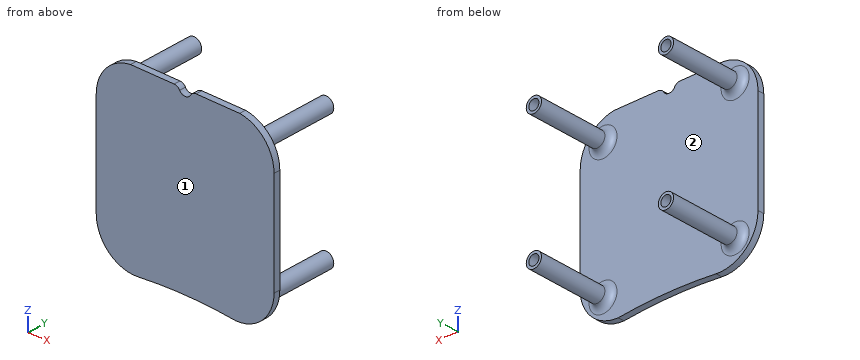
```python
from build123d import *

# Parameters (mm, degrees)
BOSS_EXTRUDE1_DEPTH = 5
SKETCH3_R           = 6
SKETCH3_R_2         = 2
BOSS_EXTRUDE2_DEPTH = 60
SKETCH4_R           = 4
CUT_EXTRUDE2_DEPTH  = 20
FILLET1_R           = 5
SKETCH5_R           = 5
CUT_EXTRUDE3_DEPTH  = 10
FILLET2_R           = 5


with BuildPart() as part:
    # Sketch2 → Boss-Extrude1 (new body)
    with BuildSketch(Plane(origin=(0, 0, 0), x_dir=(1, 0, 0), z_dir=(0, 1, 0))):
        with BuildLine():
            Line((-53.508823352, -72.096737708), (32.436645713, -72.096737708))
            ThreePointArc((32.436645713, -72.096737708), (51.703313555, -62.379157363), (59.46391118, -42.24438689))
            Line((59.46391118, -42.24438689), (59.46391118, 38.050911473))
            ThreePointArc((59.46391118, 38.050911473), (50.695521882, 59.245691656), (29.51599738, 68.050866257))
            ThreePointArc((29.51599738, 68.050866257), (-9.019885151, 65.996186888), (-47.563354288, 67.903262292))
            ThreePointArc((-47.563354288, 67.903262292), (-70.670859293, 60.290313848), (-80.53608882, 38.050911473))
            Line((-80.53608882, 38.050911473), (-80.53608882, -42.24438689))
            ThreePointArc((-80.53608882, -42.24438689), (-72.775491194, -62.379157363), (-53.508823352, -72.096737708))
        make_face()
    extrude(amount=BOSS_EXTRUDE1_DEPTH)

    # Sketch3 → Boss-Extrude2 (add)
    # profile 1 of 4: a face of its own
    with BuildSketch(Plane(origin=(0, 5, 0), x_dir=(1, 0, 0), z_dir=(0, 1, 0))):
        with Locations(Location((41.46391118, 49.903262292, 0), (0, 0, 90))):
            Circle(SKETCH3_R)
        with Locations(Location((41.46391118, 49.903262292, 0), (0, 0, 270))):
            Circle(SKETCH3_R_2, mode=Mode.SUBTRACT)
    # profile 2 of 4: a face of its own
    with BuildSketch(Plane(origin=(0, 5, 0), x_dir=(1, 0, 0), z_dir=(0, 1, 0))):
        with Locations(Location((-62.53608882, 49.903262292, 0), (0, 0, 90))):
            Circle(SKETCH3_R)
        with Locations(Location((-62.53608882, 49.903262292, 0), (0, 0, 90))):
            Circle(SKETCH3_R_2, mode=Mode.SUBTRACT)
    # profile 3 of 4: a face of its own
    with BuildSketch(Plane(origin=(0, 5, 0), x_dir=(1, 0, 0), z_dir=(0, 1, 0))):
        with Locations(Location((-62.53608882, -54.096737708, 0), (0, 0, 90))):
            Circle(SKETCH3_R)
        with Locations(Location((-62.53608882, -54.096737708, 0), (0, 0, 270))):
            Circle(SKETCH3_R_2, mode=Mode.SUBTRACT)
    # profile 4 of 4: a face of its own
    with BuildSketch(Plane(origin=(0, 5, 0), x_dir=(1, 0, 0), z_dir=(0, 1, 0))):
        with Locations(Location((41.46391118, -54.096737708, 0), (0, 0, 90))):
            Circle(SKETCH3_R)
        with Locations(Location((41.46391118, -54.096737708, 0), (0, 0, 90))):
            Circle(SKETCH3_R_2, mode=Mode.SUBTRACT)
    extrude(amount=BOSS_EXTRUDE2_DEPTH)

    # Sketch4 → Cut-Extrude2 (cut)
    with BuildSketch(Plane(origin=(0, 65, 0), x_dir=(1, 0, 0), z_dir=(0, 1, 0))):
        with Locations(Location((41.46391118, 49.903262292, 0), (0, 0, 270))):
            Circle(SKETCH4_R)
        with Locations(Location((-62.53608882, 49.903262292, 0), (0, 0, 270))):
            Circle(SKETCH4_R)
        with Locations(Location((-62.53608882, -54.096737708, 0), (0, 0, 270))):
            Circle(SKETCH4_R)
        with Locations(Location((41.46391118, -54.096737708, 0), (0, 0, 270))):
            Circle(SKETCH4_R)
    extrude(amount=-CUT_EXTRUDE2_DEPTH, mode=Mode.SUBTRACT)

    # Fillet1
    fillet1_edges = [part.edges().sort_by_distance(p)[0] for p in [
        (41.46391118, 5, -43.903262292),
        (-62.53608882, 5, -43.903262292),
        (-62.53608882, 5, 60.096737708),
        (41.46391118, 5, 60.096737708),
    ]]
    fillet(fillet1_edges, radius=FILLET1_R)

    # Sketch5 → Cut-Extrude3 (cut)
    with BuildSketch(Plane(origin=(0, 5, 0), x_dir=(1, 0, 0), z_dir=(0, 1, 0))):
        with Locations((-10.53608882, -72.096737708)):
            Circle(SKETCH5_R)
    extrude(amount=-CUT_EXTRUDE3_DEPTH, mode=Mode.SUBTRACT)

    # Fillet2
    fillet2_edges = [part.edges().sort_by_distance(p)[0] for p in [
        (-15.53608882, 2.5, 72.096737708),
        (-5.53608882, 2.5, 72.096737708),
    ]]
    fillet(fillet2_edges, radius=FILLET2_R)


solid = part.part
```
Design review of the part built by this model. Coordinates are the model's own, in mm. Face numbers are marked on the shaded views. Give positions to 0.01 mm unless a question says otherwise; leave off trailing zeros. Order: outer loops, then holes, each group sorted by start corner. A loop starts at its lowest first (then second) coordinate and runs counter-clockwise, first axis right, second up. Notation, with made-up numbers: (81.5, 60) -> (93.5, 60) arc R13 ccw to (93.5, 77) -> close; hole circle Ø10 at (-7.5, 62.5). An arc over 180 degrees is marked (long way). Write each question's results on one line, items separated by ' | '. Start each with the question number.
Q1. Wall thickness on L1, parallel to X at y = 11.5, z = -50; L2, parallel to X at y = 16.5, z = 53 (3 decimals); L3, parallel to Y at x = 27, z = -41: over which ranges is each line inside the solid? List them lowest first. Write a range as from..to.
Q2. Add section D-D on x = -44. Give the boundary of the cut face in (y, z), and give its area (3 significant figures).
Q3. For pin 1 (2 mm diameter, centred on y = 7.5, z = -15, fed in from -X); pin 2 (8 mm diameter, centred on x = -40, z = -29.5, fed in from +Y); pin 3 (3 mm diameter, centred on x = 40.5, z = -51, fed in from +Y), all flat-tipped, find the tip position at first contact; note any pin that passes through.
Q4. Add section B-B on y = 47.5. Give the boundary of the cut face in (x, z).
Q5. Add section A-A on y = 38. Give the boundary of the cut face in (x, z), and give its area (3 significant figures).
Q6. Add section C-C on z = 15. Give the boundary of the cut face in (x, y).
Q7. Mouldability with a two-part tool opening along X and no side actions: class the marked faces 1 and 2 as +X half, -X half, draft (parallel to the pull), parting line (faces both ways), or undercut.
Found:
1) L1: x = -68.54..-64.53, -60.54..-56.54, 35.46..39.47, 43.46..47.46 | L2: x = -68.435..-64.209, -60.864..-56.637, 35.565..39.791, 43.136..47.363 | L3: y = 0..5
2) outline: (0, -67.56) -> (5, -67.56) -> (5, 72.1) -> (0, 72.1) -> close | area: 698 mm2
3) pin 1: passes through | pin 2: stops at y = 5 | pin 3: stops at y = 45
4) outline: circle Ø12 at (-62.54, -49.9); circle Ø12 at (-62.54, 54.1); circle Ø12 at (41.46, -49.9); circle Ø12 at (41.46, 54.1); hole circle Ø8 at (-62.54, -49.9); hole circle Ø8 at (-62.54, 54.1); hole circle Ø8 at (41.46, -49.9); hole circle Ø8 at (41.46, 54.1)
5) outline: circle Ø12 at (-62.54, -49.9); circle Ø12 at (-62.54, 54.1); circle Ø12 at (41.46, -49.9); circle Ø12 at (41.46, 54.1); hole circle Ø4 at (-62.54, -49.9); hole circle Ø4 at (-62.54, 54.1); hole circle Ø4 at (41.46, -49.9); hole circle Ø4 at (41.46, 54.1) | area: 402 mm2
6) outline: (-80.54, 0) -> (59.46, 0) -> (59.46, 5) -> (-80.54, 5) -> close
7) face 1: draft | face 2: undercut
